Autodesk Inventor part; units mm, degrees
ref_plane "Work Plane1" through (0, 0, 0) normal (0, 0, 1) x (1, 0, 0)
ref_plane "YZ Plane" through (0, 0, 0) normal (1, 0, 0) x (0, 1, 0)
ref_plane "XZ Plane" through (0, 0, 0) normal (0, 1, 0) x (-1, 0, 0)
sketch "Sketch1" plane through (0, 0, 0) normal (0, 0, 1) x (1, 0, 0)
  line L0 (0, 0) -> (50, 0)
  line L1 (50, 0) -> (50, 5)
  line L2 (50, 5) -> (0, 5)
  line L3 (0, 5) -> (0, 0)
  dimension "d0" = 50
  dimension "d1" = 5
extrude "Extrusion1" add sketch "Sketch1" along normal blind 955
ref_plane "Work Plane1" through (0, 0, 0) normal (0, 0, 1) x (1, 0, 0)
sketch "Sketch3" plane through (0, 0, 0) normal (0, 0, 1) x (1, 0, 0)
  line L0 (0, 0) -> (50, 0)
  line L1 (0, 5) -> (0, 0)
  line L2 (50, 5) -> (0, 5)
  line L3 (50, 0) -> (50, 5)
  line L4 (0, 5) -> (50, 5)
  line L5 (0, 5) -> (0, 25)
  line L6 (50, 25) -> (0, 25)
  line L7 (50, 5) -> (50, 25)
sketch "Sketch5" plane through (0, 5, 0) normal (0, 1, 0) x (1, 0, 0)
  line L0 (70, -440) -> (70, -460)
  line L1 (-20, -440) -> (-20, -460)
  line L2 (50, 0) -> (0, 0)
  line L3 (-20, -460) -> (70, -460)
  line L4 (-20, -440) -> (70, -440)
  point P0 (50, -450)
  dimension "d33" = 20
extrude "Extrusion7" add sketch "Sketch5" along normal blind 20
sketch "Sketch7" plane through (70, 5, 460) normal (1, 0, 0) x (0, 0, -1)
  circle A0 centre (10, 10) radius 5
  point P0 (460, -5)
  dimension "d39" = 10
extrude "Extrusion8" cut sketch "Sketch7" against normal blind 100
Source: CAD feature listing. Evaluate the final solid. Frame: model axes, mm. A direction names the side the tool comes from. Give positions to 0.01 mm unless a question says otherwise; leave off trailing zeros. Loops run counter-clockwise (first coordinate to the right, second up) from the corner with the lowest first, then second, coordinate; pieces in that order, holes last. Notation, with made-up numbers: (37, 23.25) - (66, 23.25) arc R24 cw to (66, 36.25) - close; hole circle Ø10 at (-23, 51). An arc over 180 degrees is marked (long way). Use CSV: the item, a comma, the result in double quotes. Start each with the question number.
1. Ray query, L1, parallel to Y at x = 11, z = 450; L2, parallel to Z at x = 46, y = 14.75; L3, parallel to Z at x = 37, y = 20.5. Return the intervals inside material, ascending.
2. Section D-D (x = 58). Output: boundary loops of the cut face in (y, z), then the cut area to 3 significant figures.
3. Section B-B (x = 8.5). Output: boundary loops of the cut face in (y, z), then the cut area to 3 significant figures.
4. Section A-A (y = 15). Output: boundary loops of the cut face in (x, z), then the cut area to 3 significant figures.
5. Section C-C (z = 795.5). Output: boundary loops of the cut face in (x, y).
6. Reachability of faces 1 (the flat face through (-10, 5, 450)), 2 (the flat face through (60, 5, 450)), 3 (the flat face through (24, 25, 450)), 4 (the flat face through (25, 5, 217)), 5 (the flat face through (25, 5, 704)) from +Z, -Z, +X, -X, +Y, -Y: full face, straight path, thin tool, end or side. Return the list, or none.
7. Pin query (flat end, axial travel): pin 1 (2.5 mm diameter, centred on y = 2, z = 556, fed in from +X); pin 2 (10 mm diameter, centred on x = -9, z = 445.5, fed in from -Y); pin 3 (6 mm diameter, centred on x = 29.5, y = 5.5, fed in from +Z); pin 4 (4 mm diameter, centred on y = 8.5, z = 187.5, fed in from -X). Return the tip coordinate at first contact, or that it passes through.
Response:
1,L1,"0 to 10, 20 to 25"
1,L2,"440 to 445.01, 454.99 to 460"
1,L3,"440 to 460"
2,outline,"(5, 440) - (25, 440) - (25, 460) - (5, 460) - close; hole circle Ø10 at (15, 450)"
2,area,"321 mm²"
3,outline,"(0, 0) - (5, 0) - (5, 440) - (25, 440) - (25, 460) - (5, 460) - (5, 955) - (0, 955) - close; hole circle Ø10 at (15, 450)"
3,area,"5,100 mm²"
4,outline,"(-20, 440) - (70, 440) - (70, 445) - (-20, 445) - close; (-20, 455) - (70, 455) - (70, 460) - (-20, 460) - close"
4,area,"900 mm²"
5,outline,"(0, 0) - (50, 0) - (50, 5) - (0, 5) - close"
6,face 1,"+Z, -Z, -X, -Y"
6,face 2,"+Z, -Z, +X, -Y"
6,face 3,"+Z, -Z, +X, -X, +Y"
6,face 4,"-Z, +X, -X, +Y"
6,face 5,"+Z, +X, -X, +Y"
7,pin 1,"x = 50"
7,pin 2,"y = 5"
7,pin 3,"z = 955"
7,pin 4,"through"
